Source: CAD feature listing. Evaluate the final solid. Frame: model axes, mm. A direction names the side the tool comes from. Round coordinates to 2 decimals unless told otherwise and drop trailing zeros. Order: outer loops, then holes, each group sorted by start corner. A loop starts at its lowest first (then second) coordinate and runs counter-clockwise, first axis right, second up. Notation, with made-up numbers: (-0.75, 76) - (8.25, 76) arc R27 ccw to (8.25, 103) - close; hole circle Ø3 at (10.25, 86). An arc over 180 degrees is marked (long way). Use one line per item in the form item = value. Start each with the question number.
Q1. Draft query along Y for faces 1 (the flat face through (481.241, 120.595, 1.565)), 2 (the flat face through (-482.581, 119.452, 1.565)), 3 (the flat face through (-11, 5, 0)). Return one class per face: released by +Y, released by -Y, zero draft, split by the parting line, or undercut.
Q2. Cut plane B-B, the plane z = 1.55. Give the number of separate pieces and of enclosed holes in the cut face, and give its area (3 significant figures).
Q3. Pin query (flat end, axial travel): pin 1 Ø6.5 at (x, y) = (-536.575, -44.45) entering from -Z. Return the tip coordinate at first contact, or that it passes through.
Q4. Set-up query: faces 4 (the flat face through (-473.31, 110.596, 1.565)), 5 (the flat face through (-11, 5, 3.175)). Return all of +Z, -Z, +X, -X, +Y, -Y with unobstructed straight access to the full face (end or side cutting, diameter ignored); none if empty.
Q5. Cut plane A-A, the plane x = 453. Return the cut outline in (y, z) (3 decimals).
Q6. Ray query, line 1 (Y direction, x = -59, z = 1.4); line 2 (X direction, y = 282, z = 2.35); line 3 (X direction, y = 202.5, z = 0.15). Return the intervals inside material, ascending. Write a range as [from, to].
from build123d import *

# Parameters (mm, degrees)
SKETCH1_R              = 5.3578125
BOSS_EXTRUDE1_DEPTH    = 3.175
SKETCH2_R              = 5.3578125
CUT_EXTRUDE1_DEPTH     = 872.830950142
CUT_EXTRUDE2_DEPTH     = 872.830950142
FILLET1_R              = 3.175
F_1_1_DIAMETER_HOLE1_D = 25.4


with BuildPart() as part:
    # Sketch1 → Boss-Extrude1 (new body)
    with BuildSketch(Plane.XY):
        Polygon((781.05, 387.35), (-781.05, 387.35), (-781.05, -387.35), (-628.65, -387.35), (-628.65, -342.9), (-501.65, -342.9), (-501.65, -387.35), (501.65, -387.35), (501.65, -342.9), (628.65, -342.9), (628.65, -387.35), (781.05, -387.35), align=None)
        with Locations((-593.725, -44.45)):
            Circle(SKETCH1_R, mode=Mode.SUBTRACT)
        with Locations((-536.575, -44.45)):
            Circle(SKETCH1_R, mode=Mode.SUBTRACT)
        with Locations((536.575, -44.45)):
            Circle(SKETCH1_R, mode=Mode.SUBTRACT)
        with Locations((593.725, -44.45)):
            Circle(SKETCH1_R, mode=Mode.SUBTRACT)
        Polygon((-525.741660624, 69.011766046), (-533.633373454, 78.962186571), (-430.149, 161.036), (-422.25728717, 151.085579476), align=None, mode=Mode.SUBTRACT)
        with Locations((-645.795, 339.09)):
            Circle(SKETCH1_R, mode=Mode.SUBTRACT)
        with Locations((-51.435, 339.459169182)):
            Circle(SKETCH1_R, mode=Mode.SUBTRACT)
        Polygon((533.712268362, 79.061761082), (525.830130005, 69.103754509), (422.266861643, 151.077993427), (430.149, 161.036), align=None, mode=Mode.SUBTRACT)
        with Locations((51.435, 339.338450694)):
            Circle(SKETCH1_R, mode=Mode.SUBTRACT)
        with Locations((645.795, 339.09)):
            Circle(SKETCH1_R, mode=Mode.SUBTRACT)
    extrude(amount=BOSS_EXTRUDE1_DEPTH)

    # Sketch2 → Cut-Extrude1 (cut, through all)
    with BuildSketch(Plane.XY.offset(3.175)):
        with Locations((-313.055, 258.318)):
            Circle(SKETCH2_R)
        with Locations((-292.227, 234.354341765)):
            Circle(SKETCH2_R)
        with Locations((-690.753, -42.672)):
            Circle(SKETCH2_R)
        with Locations((-671.703, -68.072)):
            Circle(SKETCH2_R)
        with Locations((292.227, 234.354341765)):
            Circle(SKETCH2_R)
        with Locations((313.055, 258.318)):
            Circle(SKETCH2_R)
        with Locations((690.753, -42.672)):
            Circle(SKETCH2_R)
        with Locations((671.703, -68.072)):
            Circle(SKETCH2_R)
    extrude(amount=-CUT_EXTRUDE1_DEPTH, mode=Mode.SUBTRACT)

    # Sketch3 → Cut-Extrude2 (cut, through all)
    with BuildSketch(Plane.XY.offset(3.175)):
        with BuildLine():
            Line((-64.135, 321.679169182), (-38.735, 321.679169182))
            ThreePointArc((-38.735, 321.679169182), (-26.035, 308.979169182), (-38.735, 296.279169182))
            Line((-38.735, 296.279169182), (-64.135, 296.279169182))
            ThreePointArc((-64.135, 296.279169182), (-76.835, 308.979169182), (-64.135, 321.679169182))
        make_face()
        with BuildLine():
            Line((38.735, 321.679169182), (64.135, 321.679169182))
            ThreePointArc((64.135, 321.679169182), (76.835, 308.979169182), (64.135, 296.279169182))
            Line((64.135, 296.279169182), (38.735, 296.279169182))
            ThreePointArc((38.735, 296.279169182), (26.035, 308.979169182), (38.735, 321.679169182))
        make_face()
        with BuildLine():
            Line((-350.556019335, 283.378351904), (-330.943397226, 299.518520862))
            ThreePointArc((-330.943397226, 299.518520862), (-313.067001693, 297.782294287), (-314.803228268, 279.905898753))
            Line((-314.803228268, 279.905898753), (-334.415850377, 263.765729795))
            ThreePointArc((-334.415850377, 263.765729795), (-352.292245911, 265.50195637), (-350.556019335, 283.378351904))
        make_face()
        with BuildLine():
            Line((-290.735192784, 212.55542181), (-271.122570675, 228.695590768))
            ThreePointArc((-271.122570675, 228.695590768), (-253.246175141, 226.959364193), (-254.982401716, 209.082968659))
            Line((-254.982401716, 209.082968659), (-274.595023825, 192.9427997))
            ThreePointArc((-274.595023825, 192.9427997), (-292.471419359, 194.679026276), (-290.735192784, 212.55542181))
        make_face()
        with BuildLine():
            Line((-727.880738371, -17.075495686), (-708.045418559, -1.20980667))
            ThreePointArc((-708.045418559, -1.20980667), (-690.194914145, -3.194622068), (-692.179729543, -21.045126482))
            Line((-692.179729543, -21.045126482), (-712.015049355, -36.910815498))
            ThreePointArc((-712.015049355, -36.910815498), (-729.865553769, -34.9260001), (-727.880738371, -17.075495686))
        make_face()
        with BuildLine():
            Line((-670.202475675, -89.639847242), (-650.367155863, -73.774158225))
            ThreePointArc((-650.367155863, -73.774158225), (-632.516651449, -75.758973623), (-634.501466846, -93.609478037))
            Line((-634.501466846, -93.609478037), (-654.336786658, -109.475167053))
            ThreePointArc((-654.336786658, -109.475167053), (-672.187291072, -107.490351656), (-670.202475675, -89.639847242))
        make_face()
        with BuildLine():
            Line((334.54998107, 297.254089706), (353.197796006, 280.008249683))
            ThreePointArc((353.197796006, 280.008249683), (353.898783462, 262.061422203), (335.951955982, 261.360434746))
            Line((335.951955982, 261.360434746), (317.304141046, 278.60627477))
            ThreePointArc((317.304141046, 278.60627477), (316.60315359, 296.553102249), (334.54998107, 297.254089706))
        make_face()
        with BuildLine():
            Line((272.680669675, 228.213187181), (291.328484611, 210.967347158))
            ThreePointArc((291.328484611, 210.967347158), (292.029472067, 193.020519678), (274.082644588, 192.319532222))
            Line((274.082644588, 192.319532222), (255.434829652, 209.565372245))
            ThreePointArc((255.434829652, 209.565372245), (254.733842195, 227.512199725), (272.680669675, 228.213187181))
        make_face()
        with BuildLine():
            Line((650.872852602, -74.669223611), (671.187893449, -89.915833575))
            ThreePointArc((671.187893449, -89.915833575), (673.722108891, -107.69665898), (655.941283485, -110.230874422))
            Line((655.941283485, -110.230874422), (635.626242638, -94.984264458))
            ThreePointArc((635.626242638, -94.984264458), (633.092027197, -77.203439053), (650.872852602, -74.669223611))
        make_face()
        with BuildLine():
            Line((705.207416511, 0.46801413), (725.522457358, -14.778595833))
            ThreePointArc((725.522457358, -14.778595833), (728.0566728, -32.559421239), (710.275847395, -35.09363668))
            Line((710.275847395, -35.09363668), (689.960806548, -19.847026717))
            ThreePointArc((689.960806548, -19.847026717), (687.426591106, -2.066201311), (705.207416511, 0.46801413))
        make_face()
    extrude(amount=-CUT_EXTRUDE2_DEPTH, mode=Mode.SUBTRACT)

    # Fillet1
    fillet1_edges = [part.edges().sort_by_distance(p)[0] for p in [
        (430.149, 161.036, 1.5875),
        (422.266861643, 151.077993427, 1.5875),
        (525.830130005, 69.103754509, 1.5875),
        (533.712268362, 79.061761082, 1.5875),
        (-501.65, -387.35, 1.5875),
        (-501.65, -342.9, 1.5875),
        (-628.65, -342.9, 1.5875),
        (-628.65, -387.35, 1.5875),
        (-781.05, -387.35, 1.5875),
        (-781.05, 387.35, 1.5875),
        (781.05, 387.35, 1.5875),
        (781.05, -387.35, 1.5875),
        (628.65, -387.35, 1.5875),
        (628.65, -342.9, 1.5875),
        (501.65, -342.9, 1.5875),
        (501.65, -387.35, 1.5875),
        (-533.633373454, 78.962186571, 1.5875),
        (-525.741660624, 69.011766046, 1.5875),
        (-422.25728717, 151.085579476, 1.5875),
        (-430.149, 161.036, 1.5875),
    ]]
    fillet(fillet1_edges, radius=FILLET1_R)

    # 1 (1) Diameter Hole1 (through all)
    with Locations(Plane.XY.offset(3.175)):
        with Locations((-565.15, 266.7), (565.15, 266.7)):
            Hole(F_1_1_DIAMETER_HOLE1_D / 2)


solid = part.part
Completed:
q1.face_1 = undercut
q1.face_2 = undercut
q1.face_3 = zero draft
q2.separate_pieces = 1
q2.enclosed_holes = 30
q2.area = 1,180,000 mm2
q3.pin_1 = through
q4.face_4 = +Z, -Z
q4.face_5 = +Z, +X, -X, +Y, -Y
q5.outline = (-387.35, 0) - (126.752, 0) - (126.752, 3.175) - (-387.35, 3.175) - close; (142.949, 0) - (387.35, 0) - (387.35, 3.175) - (142.949, 3.175) - close
q6.line_1 = [-387.35, 296.28], [321.68, 387.35]
q6.line_2 = [-781.05, -351.99], [-312.78, 314.7], [351.04, 781.05]
q6.line_3 = [-781.05, -295.36], [-262.98, 263.07], [295.38, 781.05]
